Input: part model. Units: mm. Frame: model coordinates. A direction names the side the tool comes from. Coordinates: 2 decimals unless noted, no trailing zeros. Loops run counter-clockwise (first coordinate to the right, second up) from the corner with the lowest first, then second, coordinate; pieces in that order, holes last. Notation, with made-up numbers: M 65,45.25 L 96,45.25 A14 ccw 96,49.25 Z; hole C 36.5,28 d3. An arc over 180 degrees is marked long. Use a Markdown table: item, result. Add a question column.
1. Line query: L1, parallel to Y at x = 0, z = 64; L2, parallel to Z at x = -18, y = -2; L3, parallel to Y at x = 8, z = 67.5. Output: solid intervals per line, ascending. Write a range as [from, to].
2. Draft query along Z for faces 6 (the cylindrical face through (19.8, 6.2, -2.3)), 7 (the flat face through (-11.9, -13.4, -8)), 8 (the cylindrical face through (-2.75, 12.4, 147.46)), 9 (the flat face through (-7, -20, 0)). Return one class per face: +Z half, -Z half, draft (parallel to the pull), parting line (faces both ways), or undercut.
3. Section C-C on z = 65. Output: boundary loops of the cut face in (x, y), then the cut area to 3 significant figures.
4. Pin query (flat end, axial travel): pin 1 (1.5 mm diameter, centred on x = -9, z = 37.5, fed in from -Y); pin 2 (5 mm diameter, centred on y = 6, z = 97.5, fed in from -X); pin 3 (8 mm diameter, centred on y = -21.5, z = 72, fed in from +X). Return the tip coordinate at first contact, or that it passes through.
5. Set-up query: faces 1 (the cylindrical face through (-3.848, 17.328, 64.964)), 2 (the flat face through (11.23, -4.64, 150)), 3 (the cylindrical face through (-11.99, -0.53, 144.93)), 4 (the flat face through (13, 0, 145)), 5 (the conical face through (-4.53, 20.38, -4.88)). Return all of +Z, -Z, +X, -X, +Y, -Y with unobstructed straight access to the full face (end or side cutting, diameter ignored); none if empty.
6. Section A-A on y = 0. Output: boundary loops of the cut face in (x, z).
Autodesk Inventor part; units mm, degrees
ref_plane "YZ Plane" through (0, 0, 0) normal (1, 0, 0) x (0, 1, 0)
ref_plane "XZ Plane" through (0, 0, 0) normal (0, 1, 0) x (-1, 0, 0)
ref_plane "XY Plane" through (0, 0, 0) normal (0, 0, 1) x (1, 0, 0)
sketch "Sketch1" plane through (0, 0, 0) normal (0, 0, 1) x (1, 0, 0)
  circle A0 centre (0, 0) radius 17.75
  circle A1 centre (0, 0) radius 30
  dimension "d0" = 35.5
  dimension "d1" = 60
extrude "Extrusion1" add sketch "Sketch1" along normal blind 140
sketch "Sketch2" plane through (0, 0, 0) normal (0, 0, -1) x (-1, 0, 0)
  point P0 (0, 0)
sketch "Sketch3" plane through (0, 0, 0) normal (0, 1, 0) x (-1, 0, 0)
  line L0 (0, -10.8) -> (0, 8.8) construction
  line L1 (-30.85, 0) -> (25.85, 0) construction
  line L2 (-17.75, 140) -> (17.75, 140) construction
  line L3 (17.75, 0) -> (-17.75, 0) construction
  line L4 (-17.75, 0) -> (-17.75, -8)
  line L5 (-17.75, -8) -> (-22.75, -8)
  line L6 (-22.75, -8) -> (-22.75, -6.75)
  line L7 (-17.75, 0) -> (-20.75, 0)
  line L8 (-22.75, -6.75) -> (-20.75, -4.75)
  line L9 (-22.75, -6.75) -> (-19.9216, -6.75) construction
  line L10 (-20.75, -4.75) -> (-20.75, 0)
  point P0 (0, 0)
  dimension "d4" = 8
  dimension "d5" = 5
  dimension "d6" = 1.25
  dimension "d7" = 3
  dimension "d8" = 45
revolve "Revolution1" add sketch "Sketch3" angle 360 about axis through (0, 0, 0) along (0, 0, 1)
sketch "Sketch5" plane through (0, 0, 140) normal (0, 0, 1) x (1, 0, 0)
  circle A0 centre (0, 0) radius 12
  circle A1 centre (0, 0) radius 30
  dimension "d22" = 24
extrude "Extrusion2" add sketch "Sketch5" along normal blind 5
sketch "Sketch6" plane through (0, 0, 145) normal (0, 0, 1) x (1, 0, 0)
  circle A0 centre (0, 0) radius 12
  circle A1 centre (0, 0) radius 12.7
  dimension "d25" = 25.4
extrude "Extrusion3" add sketch "Sketch6" along normal blind 5
chamfer "Chamfer1" distance 10 angle 45 1 edges at (-30, 0, 145)
properties part number "MVX-TL and MVX-TV1X-coarse-reference"
Answers below:
| question | item | result |
|---|---|---|
| 1 | L1 | y = [-30, -17.75], [17.75, 30] |
| 1 | L2 | z = [-8, 145] |
| 1 | L3 | y = [-28.91, -15.84], [15.84, 28.91] |
| 2 | face 6 | undercut |
| 2 | face 7 | -Z half |
| 2 | face 8 | draft |
| 2 | face 9 | undercut |
| 3 | outline | C 0,0 d60; hole C 0,0 d35.5 |
| 3 | area | 1,840 mm² |
| 4 | pin 1 | stops at y = -28.84 |
| 4 | pin 2 | stops at x = -29.8 |
| 4 | pin 3 | stops at x = 24.37 |
| 5 | face 1 | -Z |
| 5 | face 2 | +Z, +X, -X, +Y, -Y |
| 5 | face 3 | +Z, -Z |
| 5 | face 4 | +Z |
| 5 | face 5 | none |
| 6 | outline | M -30,0 L -20.75,0 L -20.75,-4.75 L -22.75,-6.75 L -22.75,-8 L -17.75,-8 L -17.75,140 L -12,140 L -12,150 L -12.7,150 L -12.7,145 L -20,145 L -30,135 Z; M 12,140 L 17.75,140 L 17.75,-8 L 22.75,-8 L 22.75,-6.75 L 20.75,-4.75 L 20.75,0 L 30,0 L 30,135 L 20,145 L 12.7,145 L 12.7,150 L 12,150 Z |
